from build123d import *

# Parameters (mm, degrees)
SKETCH1_W               = 3.175
SKETCH1_H               = 20
BOSS_EXTRUDE1_DEPTH     = 3.175
CUT_EXTRUDE1_DEPTH      = 154.72662678
CUT_EXTRUDE1_DEPTH_BACK = 154.72662678
SKETCH2_R               = 1.6
CUT_EXTRUDE2_DEPTH      = 154.72662678
CUT_EXTRUDE2_DEPTH_BACK = 154.72662678
SKETCH3_R               = 1.6


with BuildPart() as part:
    # Sketch1 → Boss-Extrude1 (new body)
    with BuildSketch(Plane(origin=(0, 0, 0), x_dir=(1, 0, 0), z_dir=(0, 1, 0))):
        with BuildLine():
            Line((-14.5875, 0), (-14.5875, -140))
            ThreePointArc((-14.5875, -140), (-1.5875, -153), (11.4125, -140))
            Line((11.4125, -140), (11.4125, 0))
            Line((11.4125, 0), (0, 0))
            Line((0, 0), (0, -80))
            Line((0, -80), (-3.175, -80))
            Line((-3.175, -80), (-3.175, 0))
            Line((-3.175, 0), (-14.5875, 0))
        make_face()
        with Locations((-1.5875, -98)):
            Rectangle(SKETCH1_W, SKETCH1_H, mode=Mode.SUBTRACT)
    extrude(amount=BOSS_EXTRUDE1_DEPTH)

    # Sketch2 → Cut-Extrude1 (cut, two sides: drawn at the far end of the back side and taken through both)
    with BuildSketch(Plane(origin=(0, 3.175, 0), x_dir=(1, 0, 0), z_dir=(0, 1, 0)).offset(-CUT_EXTRUDE1_DEPTH_BACK)):
        with Locations(Location((5, -135, 0), (0, 0, 270))):
            Circle(SKETCH2_R)
        with Locations(Location((-8.175, -135, 0), (0, 0, 270))):
            Circle(SKETCH2_R)
    extrude(amount=CUT_EXTRUDE1_DEPTH + CUT_EXTRUDE1_DEPTH_BACK, mode=Mode.SUBTRACT)

    # Sketch3 → Cut-Extrude2 (cut, two sides: drawn at the far end of the back side and taken through both)
    with BuildSketch(Plane(origin=(0, 3.175, 0), x_dir=(1, 0, 0), z_dir=(0, 1, 0)).offset(-CUT_EXTRUDE2_DEPTH_BACK)):
        with Locations(Location((-11.5875, -8, 0), (0, 0, 270))):
            Circle(SKETCH3_R)
        with Locations(Location((-11.5875, -3, 0), (0, 0, 270))):
            Circle(SKETCH3_R)
        with Locations(Location((8.4125, -8, 0), (0, 0, 270))):
            Circle(SKETCH3_R)
        with Locations(Location((8.4125, -3, 0), (0, 0, 270))):
            Circle(SKETCH3_R)
    extrude(amount=CUT_EXTRUDE2_DEPTH + CUT_EXTRUDE2_DEPTH_BACK, mode=Mode.SUBTRACT)


solid = part.part
The model under review builds one solid part; all positions refer to its coordinate system, in mm. A direction names the side the tool comes from. Coordinates: 2 decimals unless noted, no trailing zeros. Loops run counter-clockwise (first coordinate to the right, second up) from the corner with the lowest first, then second, coordinate; pieces in that order, holes last. Notation, with made-up numbers: (-5, -25.5) -> (29, -25.5) arc R19 cw to (29, -5.5) -> close; hole circle Ø11 at (86, 79). An arc over 180 degrees is marked (long way). Use a Markdown table: item, result. Add a question column.
1. To check wall thickness, follow line 1 (X direction, y = 1.85, z = 135) (1 decimal); line 2 (X direction, y = 1.65, z = 51) (1 decimal); line 3 (Z direction, x = -11.5, y = 1.95). State the ranges of each line that lie inside material, in increasing order.
2. Add section D-D on z = 101.5. Write out the cut boundary in (x, y) (1 decimal).
3. Add section A-A on z = 135. Write out the cut boundary in (x, y) (1 decimal), plus the area to 3 significant figures.
4. Add section B-B on z = 3. Write out the cut boundary in (x, y) (1 decimal).
5. Machinability: for faces 5 (the face through (-3.175, 2, 41)), 6 (the face through (-14.588, 2, 69)), 7 (the face through (-2, 2, 88)), which of the approach directions +Z, -Z, +X, -X, +Y, -Y give a long, thin tool a straight path to every point of the face, cutting with its end or side? Answer none if there is none.
6. Draft analysis for pull direction Z (two halves, no side actions). For faces 1 (the face through (10, 1.6, 2.8)), 2 (the face through (-8.788, 1.565, 136.478)), 3 (the face through (0, 2, 39)), 4 (the face through (6, 2, 0)), state which applies: pulls with the +Z half, pulls with the -Z half, needs draft (parallel to the pull), parting line crosses it, or undercut.
7. Clearance check with flat-ended pins moving along their axes: pin 1 Ø2.5 at (x, z) = (8.41, 8) entering from -Y; pin 2 Ø1.6 at (x, y) = (-1.5, 2) entering from -Z; pin 3 Ø1 at (x, y) = (4.5, 2) entering from +Z. State where each tip first meets the part, or that it passes through.
8. Add section C-C on x = 5. Write out the cut boundary in (y, z) (3 decimals), plus the area to 3 significant figures.
Returned:
| question | item | result |
|---|---|---|
| 1 | line 1 | x = -14.6 to -9.8, -6.6 to 3.4, 6.6 to 11.4 |
| 1 | line 2 | x = -14.6 to -3.2, 0 to 11.4 |
| 1 | line 3 | z = 0 to 1.4, 4.6 to 6.4, 9.6 to 148.41 |
| 2 | outline | (-14.6, 0) -> (-3.2, 0) -> (-3.2, 3.2) -> (-14.6, 3.2) -> close; (0, 0) -> (11.4, 0) -> (11.4, 3.2) -> (0, 3.2) -> close |
| 3 | outline | (-14.6, 0) -> (-9.8, 0) -> (-9.8, 3.2) -> (-14.6, 3.2) -> close; (-6.6, 0) -> (3.4, 0) -> (3.4, 3.2) -> (-6.6, 3.2) -> close; (6.6, 0) -> (11.4, 0) -> (11.4, 3.2) -> (6.6, 3.2) -> close |
| 3 | area | 62.2 mm² |
| 4 | outline | (-14.6, 0) -> (-13.2, 0) -> (-13.2, 3.2) -> (-14.6, 3.2) -> close; (-10, 0) -> (-3.2, 0) -> (-3.2, 3.2) -> (-10, 3.2) -> close; (0, 0) -> (6.8, 0) -> (6.8, 3.2) -> (0, 3.2) -> close; (10, 0) -> (11.4, 0) -> (11.4, 3.2) -> (10, 3.2) -> close |
| 5 | face 5 | -Z, +Y, -Y |
| 5 | face 6 | +Z, -Z, -X, +Y, -Y |
| 5 | face 7 | +Y, -Y |
| 6 | face 1 | undercut |
| 6 | face 2 | undercut |
| 6 | face 3 | needs draft |
| 6 | face 4 | pulls with the -Z half |
| 7 | pin 1 | passes through |
| 7 | pin 2 | stops at z = 80 |
| 7 | pin 3 | stops at z = 151.74 |
| 8 | outline | (0, 0) -> (3.175, 0) -> (3.175, 133.4) -> (0, 133.4) -> close; (0, 136.6) -> (3.175, 136.6) -> (3.175, 151.207) -> (0, 151.207) -> close |
| 8 | area | 470 mm² |
